from build123d import *

# Parameters (mm, degrees)
PATTERN_CIRCULAR_1_COUNT = 6


with BuildPart() as part:
    # Эскиз1 → Повернуть1 (revolve)
    with BuildSketch(Plane(origin=(0, 0, 0), x_dir=(0, 0, -1), z_dir=(1, 0, 0)), mode=Mode.PRIVATE) as revolve_1_sk:
        Polygon((0, 31), (19, 31), (19, 24), (17, 24), (17, 26), (0, 26), align=None)
    revolve(revolve_1_sk.sketch.rotate(Axis((0, 0, 0), (0, 0, -1)), 90), axis=Axis((0, 0, 0), (0, 0, -1)))

    # Эскиз3 → Сверло под метчик  спиральное M31 (revolve, cut)
    with BuildSketch(Plane(origin=(28.5, 0, 0), x_dir=(0, -1, 0), z_dir=(1, 0, 0))):
        Polygon((0, 0), (0, 8.946355475), (1.575, 8), (1.575, 0), align=None)
    hole_wizard_m31 = revolve(axis=Axis((28.5, 0, 6.35), (0, 0, -1)), mode=Mode.SUBTRACT)

    # Круговой массив1: Сверло под метчик  спиральное M31 ×6 about axis
    pattern_circular_1_axis = Axis((0, 0, 0), (0, 0, 1))
    for i in range(1, PATTERN_CIRCULAR_1_COUNT):
        add(hole_wizard_m31.rotate(pattern_circular_1_axis, i * 360 / PATTERN_CIRCULAR_1_COUNT), mode=Mode.SUBTRACT)


solid = part.part
Check sheet for the modelled part. Datum: model origin and axes. Units: mm. A direction names the side the tool comes from. Round coordinates to 2 decimals unless told otherwise and drop trailing zeros. Loops run counter-clockwise (first coordinate to the right, second up) from the corner with the lowest first, then second, coordinate; pieces in that order, holes last. Notation, with made-up numbers: M -36.75,-10 L 17.25,-10 A24 ccw 17.25,12 Z; hole C -28,50.25 d8. An arc over 180 degrees is marked long. One line per item, written item: value.
(1) Sectioned sample at D-D, the plane z = -3. Record the cut outline in (x, y) (3 decimals).
Computed values:
outline: C 0,0 d62; hole C -28.5,0 d3.15; hole C 0,0 d52; hole C -14.25,-24.682 d3.15; hole C -14.25,24.682 d3.15; hole C 14.25,-24.682 d3.15; hole C 14.25,24.682 d3.15; hole C 28.5,0 d3.15
(2) Sectioned sample at C-C, the plane z = -12.75. Record the cut outline in (x, y), then the cut area to 3 significant figures.
Computed values:
outline: C 0,0 d62; hole C 0,0 d52
area: 895 mm^2
(3) Sectioned sample at B-B, the plane y = 13.5. Record the cut outline in (x, z), then the cut area to 3 significant figures.
Computed values:
outline: M -27.91,-19 L -19.84,-19 L -19.84,-17 L -22.22,-17 L -22.22,0 L -27.91,0 Z; M 19.84,-19 L 27.91,-19 L 27.91,0 L 22.22,0 L 22.22,-17 L 19.84,-17 Z
area: 226 mm^2
(4) Release check for a two-part mould opening along Y. For faces 3 (the face through (-4.036, -30.736, -9.633)), 4 (the face through (15.9, 18.2, -19)), 5 (the face through (-14.319, 26.255, -3.944)), 6 (the face through (-14.723, -26.184, -3.944)) record: +Y half, -Y half, draft (parallel to the pull), parting line (faces both ways), or undercut.
Computed values:
face 3: parting line
face 4: draft
face 5: undercut
face 6: undercut
(5) Thickness scan on line 1 (X direction, y = 14, z = -16); line 2 (Y direction, x = 6, z = -2); line 3 (X direction, y = 6, z = -17.25). Record the ranges inside material, lowest first.
Computed values:
line 1: x = -27.66 to -21.91, 21.91 to 27.66
line 2: y = -30.41 to -25.3, 25.3 to 30.41
line 3: x = -30.41 to -23.24, 23.24 to 30.41
(6) Sectioned sample at A-A, the plane x = 0. Record the cut outline in (y, z), then the cut area to 3 significant figures.
Computed values:
outline: M -31,-19 L -24,-19 L -24,-17 L -26,-17 L -26,0 L -31,0 Z; M 24,-19 L 31,-19 L 31,0 L 26,0 L 26,-17 L 24,-17 Z
area: 198 mm^2
(7) Access from +Z, -Z, +X, -X, +Y, -Y to the whole of each face (thin tool, end or side, straight path). Record for faces 1 (the face through (22.89, -7.21, -17.99)), 2 (the face through (-30.038, -0.341, -3.944)).
Computed values:
face 1: +Z, -Z
face 2: +Z
(8) Depth check by flat-ended pin: pin 1 Ø3 at (y, z) = (15, -9) entering from -X; pin 2 Ø10 at (y, z) = (-14, -7) entering from +X; pin 3 Ø6 at (x, z) = (22, -5.5) entering from -Y. Enter the tip coordinate at first touch or a pass-through.
Computed values:
pin 1: stops at x = -27.91
pin 2: stops at x = 29.66
pin 3: stops at y = -24.49
